Build history of the part. All positions in model axes, mm. Round coordinates to 2 decimals unless told otherwise and drop trailing zeros. Write each loop counter-clockwise with the first axis right and the second up, starting at its lowest first coordinate (ties: lowest second). Pieces come first, ordered by that corner, then holes. Notation, with made-up numbers: (-13.75, 55.5) -> (23.25, 55.5) arc R20 ccw to (23.25, 73.5) -> close; hole circle Ø11 at (-22, 63.25). An arc over 180 degrees is marked (long way). Answer as CSV lines item,"result".
from build123d import *

# Parameters (mm, degrees)
SKETCH1_W           = 209
SKETCH1_H           = 107
SKETCH1_R           = 1.2
SKETCH1_W_2         = 71.3
SKETCH1_H_2         = 24.7
BOSS_EXTRUDE1_DEPTH = 3
SKETCH3_W           = 121.70473961
SKETCH3_H           = 27.18
CUT_EXTRUDE1_DEPTH  = 4
SKETCH4_W           = 12
SKETCH4_H           = 12
CUT_EXTRUDE2_DEPTH  = 4


with BuildPart() as part:
    # Sketch1 → Boss-Extrude1 (new body)
    with BuildSketch(Plane.XY):
        Rectangle(SKETCH1_W, SKETCH1_H)
        with Locations((-37.5, 11)):
            Circle(SKETCH1_R, mode=Mode.SUBTRACT)
        with Locations((37.5, 11)):
            Circle(SKETCH1_R, mode=Mode.SUBTRACT)
        with Locations((37.5, -20)):
            Circle(SKETCH1_R, mode=Mode.SUBTRACT)
        with Locations((-37.5, -20)):
            Circle(SKETCH1_R, mode=Mode.SUBTRACT)
        with Locations((0, -4.5)):
            Rectangle(SKETCH1_W_2, SKETCH1_H_2, mode=Mode.SUBTRACT)
    extrude(amount=BOSS_EXTRUDE1_DEPTH)

    # Sketch3 → Cut-Extrude1 (cut, through all)
    with BuildSketch(Plane.XY.offset(3)):
        with Locations((-0.147630195, -39.91)):
            Rectangle(SKETCH3_W, SKETCH3_H)
    extrude(amount=-CUT_EXTRUDE1_DEPTH, mode=Mode.SUBTRACT)

    # Sketch4 → Cut-Extrude2 (cut, through all)
    with BuildSketch(Plane.XY.offset(3)):
        with Locations((-51.65, -4.5)):
            Rectangle(SKETCH4_W, SKETCH4_H)
        with Locations((-73.65, -4.5)):
            Rectangle(SKETCH4_W, SKETCH4_H)
        with Locations((51.65, -4.5)):
            Rectangle(SKETCH4_W, SKETCH4_H)
    extrude(amount=-CUT_EXTRUDE2_DEPTH, mode=Mode.SUBTRACT)


solid = part.part
1. Drop flat-ended pins along their axis: pin 1 Ø2 at (x, y) = (-37.5, 11) entering from +Z; pin 2 Ø1.5 at (x, z) = (-49.5, 1.5) entering from -Y. Give the stop position or say it passes through.
Results found:
pin 1,"passes through"
pin 2,"stops at y = -26.32"
2. Cut at A-A, the plane x = 53. Write the cut outline in (y, z), then the cut area to 3 significant figures.
Results found:
outline,"(-26.32, 0) -> (-10.5, 0) -> (-10.5, 3) -> (-26.32, 3) -> close; (1.5, 0) -> (53.5, 0) -> (53.5, 3) -> (1.5, 3) -> close"
area,"203 mm2"
3. Cut at C-C, the plane x = -76. Write the cut outline in (y, z), then the cut area to 3 significant figures.
Results found:
outline,"(-53.5, 0) -> (-10.5, 0) -> (-10.5, 3) -> (-53.5, 3) -> close; (1.5, 0) -> (53.5, 0) -> (53.5, 3) -> (1.5, 3) -> close"
area,"285 mm2"
4. Cut at B-B, the plane z = 1.5. Count the separate pieces of the cut face and the enclosed holes in it, then the cut area to 3 significant figures.
Results found:
separate pieces,"1"
enclosed holes,"8"
area,"16,800 mm2"
5. Probe line 1 along Y through (x, z) = (-37.5, 2.25); line 2 along Y through (x, z) = (-79, 1.1); line 3 along X through (y, z) = (3, 0.4). List the from-to ranges inside material, lowest first.
Results found:
line 1,"y = -26.32 to -21.2, -18.8 to 9.8, 12.2 to 53.5"
line 2,"y = -53.5 to -10.5, 1.5 to 53.5"
line 3,"x = -104.5 to -35.65, 35.65 to 104.5"
